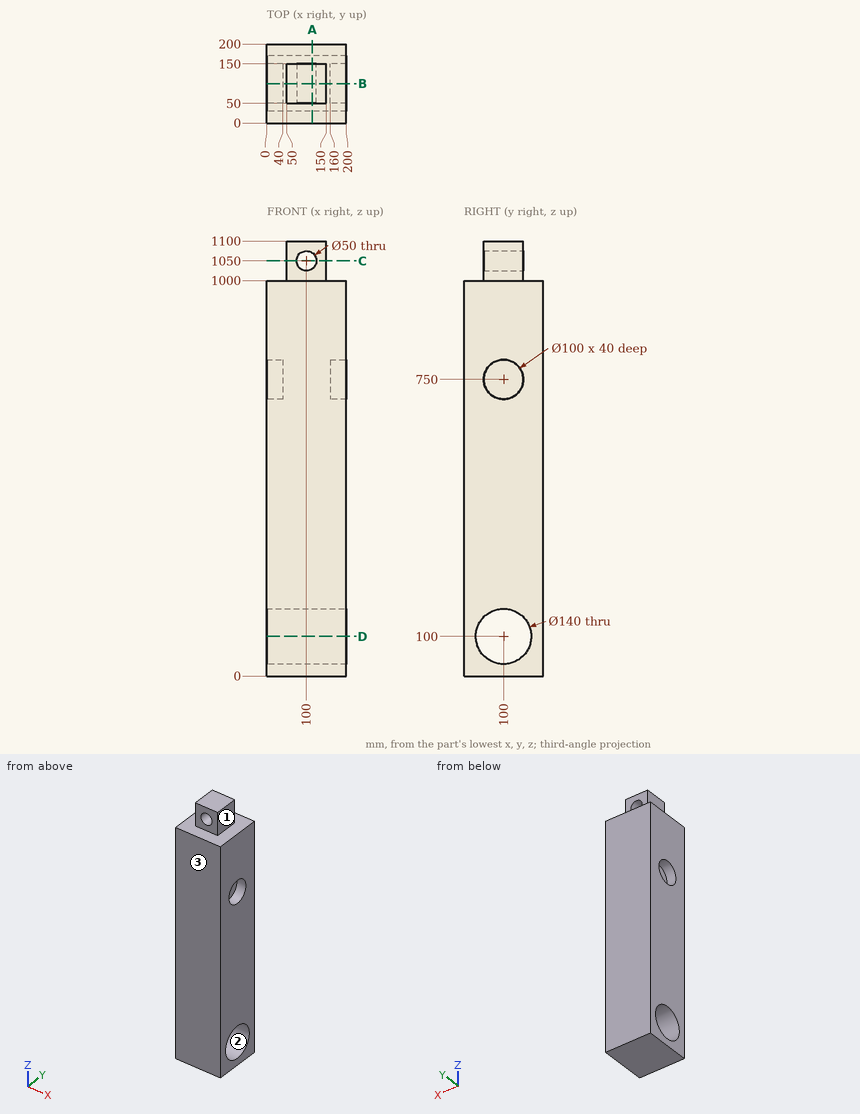
Verification items for this drawing (mm, ordinates from the low corner). Give positions to 0.01 mm unless a question says otherwise; leave off trailing zeros. Loops run counter-clockwise (first coordinate to the right, second up) from the corner with the lowest first, then second, coordinate; pieces in that order, holes last.
1. Release check for a two-part mould opening along Y. For the marked faces 1, 2 and 3 record: +Y half, -Y half, draft (parallel to the pull), parting line (faces both ways), or undercut.
Derived:
face 1: draft
face 2: undercut
face 3: -Y half
2. Material ranges on probe 1 along Z at (x, y) = (16, 104); probe 2 along Y at (x, z) = (74.5, 100); probe 3 along X at (y, z) = (125, 1050), recorded low to high.
Derived:
probe 1: z = 0 to 30.11, 169.89 to 700.16, 799.84 to 1000
probe 2: y = 0 to 30, 170 to 200
probe 3: x = 50 to 75, 125 to 150
3. Cross-section at B-B on y = 100. Record the cut outline in (x, z), and give its area (3 significant figures).
Derived:
outline: (0, 0) - (200, 0) - (200, 30) - (0, 30) - close; (0, 170) - (200, 170) - (200, 700) - (160, 700) - (160, 800) - (200, 800) - (200, 1000) - (150, 1000) - (150, 1100) - (50, 1100) - (50, 1000) - (0, 1000) - (0, 800) - (40, 800) - (40, 700) - (0, 700) - close; hole circle Ø50 at (100, 1050)
area: 172,000 mm2
4. Cross-section at C-C on z = 1050. Record the cut outline in (x, y).
Derived:
outline: (50, 50) - (75, 50) - (75, 150) - (50, 150) - close; (125, 50) - (150, 50) - (150, 150) - (125, 150) - close
5. Cross-section at A-A on x = 115. Record the cut outline in (y, z).
Derived:
outline: (0, 0) - (200, 0) - (200, 1000) - (150, 1000) - (150, 1030) - (50, 1030) - (50, 1000) - (0, 1000) - close; (50, 1070) - (150, 1070) - (150, 1100) - (50, 1100) - close; hole circle Ø140 at (100, 100)
6. Go/stop test with a flat-tipped pin: P1, Ø1.5, axis at y = 71, z = 767, coming from the +X side. Record where the tip stops, or that it passes through.
Derived:
P1: stops at x = 160
7. Cross-section at D-D on z = 100. Record the cut outline in (x, y).
Derived:
outline: (0, 0) - (200, 0) - (200, 30) - (0, 30) - close; (0, 170) - (200, 170) - (200, 200) - (0, 200) - close
